from build123d import *

# Parameters (mm, degrees)
ESQUISSE1_R                         = 15.25
ESQUISSE1_R_2                       = 13.5
BOSS_EXTRU_1_DEPTH                  = 145
ENL_V_MAT_EXTRU_1_REACH             = 148.595
ESQUISSE4_R                         = 2
ENL_V_MAT_EXTRU_1_DIRECTION_2_DEPTH = 147.595105648
ESQUISSE5_W                         = 170
ESQUISSE5_H                         = 115
BOSS_EXTRU_2_DEPTH                  = 9
ESQUISSE14_R                        = 14
ENL_V_MAT_EXTRU_2_DEPTH             = 186.060125365
ENL_V_MAT_EXTRU_3_DEPTH             = 186.060125448
ENL_V_MAT_EXTRU_3_DEPTH_BACK        = 186.060125448
ESQUISSE15_R                        = 1.5
ESQUISSE16_R                        = 1.75
ENL_V_MAT_EXTRU_4_DEPTH             = 15
ESQUISSE22_W                        = 70
ESQUISSE22_H                        = 3
BOSS_EXTRU_11_DEPTH                 = 90
ENL_V_MAT_EXTRU_6_DEPTH             = 90
ESQUISSE25_W                        = 4
ESQUISSE25_H                        = 32
ENL_V_MAT_EXTRU_7_DEPTH             = 90
ENL_V_MAT_EXTRU_8_REACH             = 187.06
ENL_V_MAT_EXTRU_8_END_RADIUS        = 15.25
ESQUISSE26_W                        = 15.960277927
ESQUISSE26_H                        = 17.240886996
ESQUISSE27_R                        = 3.25
BOSS_EXTRU_12_DEPTH                 = 12
ENL_V_MAT_EXTRU_9_DEPTH             = 178.640789317


with BuildPart() as part:
    # Esquisse1 → Boss.-Extru.1 (new body)
    with BuildSketch(Plane.XY):
        Circle(ESQUISSE1_R)
        Circle(ESQUISSE1_R_2, mode=Mode.SUBTRACT)
    extrude(amount=BOSS_EXTRU_1_DEPTH)

    # Esquisse4 → Enlèv. mat.-Extru.1 (cut, up to next)
    with BuildSketch(Plane(origin=(0, 0, 0), x_dir=(1, 0, 0), z_dir=(0, 1, 0)), mode=Mode.PRIVATE) as enl_v_mat_extru_1_sk1:
        with Locations(Location((0, -52.5, 0), (0, 0, 270))):
            Circle(ESQUISSE4_R)
    enl_v_mat_extru_1_tool1 = extrude(enl_v_mat_extru_1_sk1.sketch, amount=-ENL_V_MAT_EXTRU_1_REACH, mode=Mode.PRIVATE) & part.part
    add(enl_v_mat_extru_1_tool1.solids().sort_by_distance((0, 0, 52.5))[0], mode=Mode.SUBTRACT)

    # Esquisse4 → Enlèv. mat.-Extru.1 direction 2 (cut)
    with BuildSketch(Plane(origin=(0, 0, 0), x_dir=(1, 0, 0), z_dir=(0, 1, 0))):
        with Locations(Location((0, -52.5, 0), (0, 0, 270))):
            Circle(ESQUISSE4_R)
    extrude(amount=ENL_V_MAT_EXTRU_1_DIRECTION_2_DEPTH, mode=Mode.SUBTRACT)

    # Esquisse5 → Boss.-Extru.2 (add)
    with BuildSketch(Plane.XY.offset(145)):
        Rectangle(ESQUISSE5_W, ESQUISSE5_H)
    extrude(amount=BOSS_EXTRU_2_DEPTH)

    # Esquisse14 → Enlèv. mat.-Extru.2 (cut, through all)
    with BuildSketch(Plane.XY):
        Circle(ESQUISSE14_R)
    extrude(amount=ENL_V_MAT_EXTRU_2_DEPTH, mode=Mode.SUBTRACT)

    # Esquisse15 → Enlèv. mat.-Extru.3 (cut, two sides: drawn at the far end of the back side and taken through both)
    with BuildSketch(Plane.XY.offset(154).offset(-ENL_V_MAT_EXTRU_3_DEPTH_BACK)):
        with Locations((-63.25, 33)):
            Circle(ESQUISSE15_R)
        with Locations((63.25, 33)):
            Circle(ESQUISSE15_R)
        with Locations((63.25, -33)):
            Circle(ESQUISSE15_R)
        with Locations((-63.25, -33)):
            Circle(ESQUISSE15_R)
    extrude(amount=ENL_V_MAT_EXTRU_3_DEPTH + ENL_V_MAT_EXTRU_3_DEPTH_BACK, mode=Mode.SUBTRACT)

    # Esquisse16 → Enlèv. mat.-Extru.4 (cut)
    with BuildSketch(Plane(origin=(0, 57.5, 0), x_dir=(1, 0, 0), z_dir=(0, 1, 0))):
        with Locations(Location((0, -149.5, 0), (0, 0, 270))):
            Circle(ESQUISSE16_R)
    extrude(amount=-ENL_V_MAT_EXTRU_4_DEPTH, mode=Mode.SUBTRACT)

    # Esquisse22 → Boss.-Extru.11 (add)
    with BuildSketch(Plane(origin=(0, 0, 145), x_dir=(-1, 0, 0), z_dir=(0, 0, -1))):
        with Locations((0, 34)):
            Rectangle(ESQUISSE22_W, ESQUISSE22_H)
    extrude(amount=BOSS_EXTRU_11_DEPTH)

    # Esquisse23 → Enlèv. mat.-Extru.6 (cut)
    with BuildSketch(Plane(origin=(0, 35.5, 0), x_dir=(1, 0, 0), z_dir=(0, 1, 0))):
        with BuildLine():
            ThreePointArc((26.5, -135), (26.060660172, -133.939339828), (25, -133.5))
            Line((25, -133.5), (25, -135))
            Line((25, -135), (23.5, -135))
            ThreePointArc((23.5, -135), (25, -136.5), (26.5, -135))
        make_face()
        with BuildLine():
            Line((25, -135), (25, -133.5))
            ThreePointArc((25, -133.5), (23.939339828, -133.939339828), (23.5, -135))
            Line((23.5, -135), (25, -135))
        make_face()
        with BuildLine():
            ThreePointArc((-22.5, -135), (-22.939339828, -133.939339828), (-24, -133.5))
            Line((-24, -133.5), (-24, -135))
            Line((-24, -135), (-22.5, -135))
        make_face()
        with BuildLine():
            Line((-24, -135), (-24, -133.5))
            ThreePointArc((-24, -133.5), (-25.060660172, -136.060660172), (-22.5, -135))
            Line((-22.5, -135), (-24, -135))
        make_face()
        with BuildLine():
            ThreePointArc((26.5, -77), (25, -75.5), (23.5, -77))
            Line((23.5, -77), (25, -77))
            Line((25, -77), (25, -78.5))
            ThreePointArc((25, -78.5), (26.060660172, -78.060660172), (26.5, -77))
        make_face()
        with BuildLine():
            Line((25, -77), (23.5, -77))
            ThreePointArc((23.5, -77), (23.939339828, -78.060660172), (25, -78.5))
            Line((25, -78.5), (25, -77))
        make_face()
        with BuildLine():
            ThreePointArc((-24, -78.5), (-22.939339828, -78.060660172), (-22.5, -77))
            Line((-22.5, -77), (-24, -77))
            Line((-24, -77), (-24, -78.5))
        make_face()
        with BuildLine():
            Line((-24, -77), (-22.5, -77))
            ThreePointArc((-22.5, -77), (-25.060660172, -75.939339828), (-24, -78.5))
            Line((-24, -78.5), (-24, -77))
        make_face()
    extrude(amount=-ENL_V_MAT_EXTRU_6_DEPTH, mode=Mode.SUBTRACT)

    # Esquisse25 → Enlèv. mat.-Extru.7 (cut)
    with BuildSketch(Plane(origin=(0, 0, 145), x_dir=(-1, 0, 0), z_dir=(0, 0, -1))):
        with Locations((-52, 1.5)):
            Rectangle(ESQUISSE25_W, ESQUISSE25_H)
    extrude(amount=-ENL_V_MAT_EXTRU_7_DEPTH, mode=Mode.SUBTRACT)

    # Enlèv. mat.-Extru.8: up to this cylinder (the profile starts inside it)
    enl_v_mat_extru_8_end = Plane(origin=(0, 0, 68.486818), z_dir=(0, 0, -1)) * Cylinder(ENL_V_MAT_EXTRU_8_END_RADIUS, 405.62, mode=Mode.PRIVATE)
    # Esquisse26 → Enlèv. mat.-Extru.8 (cut, up to the surface)
    with BuildSketch(Plane(origin=(0, 0, 0), x_dir=(1, 0, 0), z_dir=(0, 1, 0)), mode=Mode.PRIVATE) as enl_v_mat_extru_8_sk1:
        with Locations((-0.793346945, -68.486817672)):
            Rectangle(ESQUISSE26_W, ESQUISSE26_H)
    enl_v_mat_extru_8_tool1 = extrude(enl_v_mat_extru_8_sk1.sketch, amount=ENL_V_MAT_EXTRU_8_REACH, mode=Mode.PRIVATE) & enl_v_mat_extru_8_end
    add(enl_v_mat_extru_8_tool1.solids().sort_by_distance((-0.793347, 0, 68.486818))[0], mode=Mode.SUBTRACT)

    # Esquisse27 → Boss.-Extru.12 (add)
    with BuildSketch(Plane.XY.offset(154)):
        with Locations((62.616003653, 32.933842855)):
            Circle(ESQUISSE27_R)
        with Locations((62.622273681, -33.123005587)):
            Circle(ESQUISSE27_R)
        with Locations((-62.800064313, -33.084450181)):
            Circle(ESQUISSE27_R)
        with Locations((-62.872546265, 32.930245113)):
            Circle(ESQUISSE27_R)
    extrude(amount=BOSS_EXTRU_12_DEPTH)

    # Esquisse29 → Enlèv. mat.-Extru.9 (cut, through all)
    with BuildSketch(Plane(origin=(0, 0, 145), x_dir=(-1, 0, 0), z_dir=(0, 0, -1))):
        with BuildLine():
            ThreePointArc((64.75, 33), (63.25, 34.5), (61.75, 33))
            Line((61.75, 33), (63.25, 33))
            Line((63.25, 33), (63.25, 31.5))
            ThreePointArc((63.25, 31.5), (64.310660172, 31.939339828), (64.75, 33))
        make_face()
        with BuildLine():
            Line((63.25, 33), (61.75, 33))
            ThreePointArc((61.75, 33), (62.189339828, 31.939339828), (63.25, 31.5))
            Line((63.25, 31.5), (63.25, 33))
        make_face()
        with BuildLine():
            ThreePointArc((64.75, -33), (64.310660172, -31.939339828), (63.25, -31.5))
            Line((63.25, -31.5), (63.25, -33))
            Line((63.25, -33), (61.75, -33))
            ThreePointArc((61.75, -33), (63.25, -34.5), (64.75, -33))
        make_face()
        with BuildLine():
            Line((63.25, -33), (63.25, -31.5))
            ThreePointArc((63.25, -31.5), (62.189339828, -31.939339828), (61.75, -33))
            Line((61.75, -33), (63.25, -33))
        make_face()
        with BuildLine():
            Line((-63.25, 31.5), (-63.25, 33))
            Line((-63.25, 33), (-61.75, 33))
            ThreePointArc((-61.75, 33), (-64.310660172, 34.060660172), (-63.25, 31.5))
        make_face()
        with BuildLine():
            Line((-61.75, 33), (-63.25, 33))
            Line((-63.25, 33), (-63.25, 31.5))
            ThreePointArc((-63.25, 31.5), (-62.189339828, 31.939339828), (-61.75, 33))
        make_face()
        with BuildLine():
            ThreePointArc((-61.75, -33), (-62.189339828, -31.939339828), (-63.25, -31.5))
            Line((-63.25, -31.5), (-63.25, -33))
            Line((-63.25, -33), (-61.75, -33))
        make_face()
        with BuildLine():
            Line((-63.25, -33), (-63.25, -31.5))
            ThreePointArc((-63.25, -31.5), (-64.310660172, -34.060660172), (-61.75, -33))
            Line((-61.75, -33), (-63.25, -33))
        make_face()
    extrude(amount=-ENL_V_MAT_EXTRU_9_DEPTH, mode=Mode.SUBTRACT)


solid = part.part
Geometry check sheet. Reference: the model listing, model coordinates, mm. A direction names the side the tool comes from. Give positions to 0.01 mm unless a question says otherwise; leave off trailing zeros. Order: outer loops, then holes, each group sorted by start corner. A loop starts at its lowest first (then second) coordinate and runs counter-clockwise, first axis right, second up. Notation, with made-up numbers: (-27.5, 75.5) - (-4.5, 75.5) arc R14 ccw to (-4.5, 85.5) - close; hole circle Ø4 at (87, -33). An arc over 180 degrees is marked (long way). Use one line per item in the form item = value.
1) Draft check along Z on faces 5 (the face through (0.088, -14.545, 50.502)), 6 (the face through (-61, -33, 166)), 7 (the face through (13.5, -4.4, 0)), 8 (the face through (0, 32.5, 101)). Enter one of: released by +Z, released by -Z, zero draft, split by the parting line, or undercut.
Working result:
face_5 = undercut
face_6 = released by +Z
face_7 = released by -Z
face_8 = zero draft
2) Access from +Z, -Z, +X, -X, +Y, -Y to the whole of each face (thin tool, end or side, straight path). Record for faces 1 (the face through (-65.2, -30.89, 159.92)), 2 (the face through (52, -14.5, 149)), 3 (the face through (-3.306, -14.887, 71.485)), 4 (the face through (0, 35.5, 101)).
Working result:
face_1 = +Z
face_2 = +Z, -Z
face_3 = -Z
face_4 = -Z, +X, -X, +Y
3) Depth check by flat-ended pin: pin 1 Ø2.5 at (y, z) = (34, 96.5) entering from +X; pin 2 Ø0.9 at (x, y) = (6.5, 34) entering from -Z; pin 3 Ø6 at (x, z) = (5.5, 81) entering from +Y; pin 4 Ø2.5 at (x, z) = (-24, 77) entering from +Y. Enter the tip coordinate at first touch or a pass-through.
Working result:
pin_1 = 35
pin_2 = 55
pin_3 = 35.5
pin_4 = through
4) Sectioned sample at D-D (y = 25.5). Record the boundary of the cut face in (x, z), and give its area (3 significant figures).
Working result:
outline = (-85, 145) - (85, 145) - (85, 154) - (-85, 154) - close
area = 1,530 mm^2
5) Sectioned sample at C-C (z = 28.5). Record the boundary of the cut face in (x, y), and give its area (3 significant figures).
Working result:
outline = circle Ø30.5 at (0, 0); hole circle Ø28 at (0, 0)
area = 115 mm^2
6) Material ranges on probe 1 along Z at (x, y) = (0, 14.85); probe 2 along Y at (x, z) = (-63, 159); probe 3 along Y at (x, z) = (0, 89), recorded low to high. Write a range as from..to.
Working result:
probe_1 = 0..50.5, 54.5..59.87, 77.11..154
probe_2 = -36.33..-34.48, -31.52..-29.84, 29.68..31.52, 34.48..36.18
probe_3 = -15.25..-14, 14..15.25, 32.5..35.5
7) Sectioned sample at A-A (z = 102). Record the boundary of the cut face in (x, y), and give its area (3 significant figures).
Working result:
outline = (-35, 32.5) - (35, 32.5) - (35, 35.5) - (-35, 35.5) - close; circle Ø30.5 at (0, 0); hole circle Ø28 at (0, 0)
area = 325 mm^2
8) Sectioned sample at B-B (x = 5). Record the boundary of the cut face in (y, z).
Working result:
outline = (-57.5, 145) - (-14.41, 145) - (-14.41, 0) - (-13.08, 0) - (-13.08, 154) - (-57.5, 154) - close; (13.08, 0) - (14.41, 0) - (14.41, 59.87) - (13.08, 59.87) - close; (13.08, 77.11) - (14.41, 77.11) - (14.41, 145) - (32.5, 145) - (32.5, 55) - (35.5, 55) - (35.5, 145) - (57.5, 145) - (57.5, 154) - (13.08, 154) - close
